from build123d import *

# Parameters (mm, degrees)
F1_DEPTH = 7.5
F3_DEPTH = 7.5
F4_SIZE  = 0.5


with BuildPart() as f1:
    # F0 (on Top) → F1 (new body, symmetric)
    with BuildSketch(Plane.XY):
        with BuildLine():
            ThreePointArc((16.7892444879, -0.9012567011), (14.177166416, 0), (16.7892444879, 0.9012567011))
            add(Edge.make_bspline(
                [(16.7892444879, 2.0751408301), (17.0817766167, 1.8643906524), (17.6043278119, 1.487926851), (17.1393225295, 0.8569863783), (16.895080973, 0.8878727844), (16.7892444879, 0.9012567011)],
                knots=[0, 0, 0, 0, 0.418834252, 0.7481651325, 1, 1, 1, 1], degree=3))
            ThreePointArc((16.7892444879, 2.0751408301), (13.2649986311, 0), (16.7892444879, -2.0751408301))
            add(Edge.make_bspline(
                [(16.7892444879, -2.0751408301), (17.0817766167, -1.8643906524), (17.6043278119, -1.487926851), (17.1393225295, -0.8569863783), (16.895080973, -0.8878727844), (16.7892444879, -0.9012567011)],
                knots=[0, 0, 0, 0, 0.418834252, 0.7481651325, 1, 1, 1, 1], degree=3))
        make_face()
    extrude(amount=F1_DEPTH, both=True)

    # F2 (on Top) → F3 (join, symmetric)
    with BuildSketch(Plane.XY):
        with BuildLine():
            ThreePointArc((11.4055118786, 1.0911012502), (12.1183137998, 0.8013586402), (12.4143324792, 0.0911401524))
            Line((12.4143324792, 0.0911401524), (12.4143324792, -0.0911401524))
            ThreePointArc((12.4143324792, -0.0911401524), (12.1183137998, -0.8013586402), (11.4055118786, -1.0911012502))
            Line((11.4055118786, -1.0911012502), (-10.2589782327, -0.9))
            Line((-10.2589782327, -0.9), (-10.2589782327, -2.1322260433))
            add(Edge.make_bspline(
                [(-10.2589782327, -2.1322260433), (-7.8308672605, -2.7680444958), (-2.1715241973, -4.4371278226), (14.2840922078, -4.2672083443), (14.5433608635, -2.4774637884), (14.5964084265, -2.1322260433)],
                knots=[0, 0, 0, 0, 0.3763600101, 0.8609680907, 1, 1, 1, 1], degree=3))
            Line((14.5964084265, -2.1322260433), (13.9306001365, -1.5301937237))
            Line((13.9306001365, -1.5301937237), (13.9306001365, 1.5301937237))
            Line((13.9306001365, 1.5301937237), (14.5964084265, 2.1322260433))
            add(Edge.make_bspline(
                [(-10.2589782327, 2.1322260433), (-7.8308672605, 2.7680444958), (-2.1715241973, 4.4371278226), (14.2840922078, 4.2672083443), (14.5433608635, 2.4774637884), (14.5964084265, 2.1322260433)],
                knots=[0, 0, 0, 0, 0.3763600101, 0.8609680907, 1, 1, 1, 1], degree=3))
            Line((-10.2589782327, 2.1322260433), (-10.2589782327, 0.9))
            Line((-10.2589782327, 0.9), (11.4055118786, 1.0911012502))
        make_face()
    extrude(amount=F3_DEPTH, both=True)

    # F4
    f4_edges = [f1.edges().sort_by_distance(p)[0] for p in [
        (-10.258978, -0.9, 0),
        (-10.258978, 0.9, 0),
    ]]
    chamfer(f4_edges, length=F4_SIZE)


solid = f1.part
Geometry check sheet. Reference: the model listing, model coordinates, mm. Give positions to 0.01 mm unless a question says otherwise; leave off trailing zeros. Answer in a Markdown table with one row per item. Add a question column.
1) Material ranges on probe 1 along Y at (x, z) = (8, -4.75); probe 2 along Y at (x, z) = (6, -3.25); probe 3 along Y at (x, z) = (12.75, -5.25), recorded low to high. Write a range as from..to.
2) Draft check along Y on faces 1 (the face through (12.11, 0.81, 0.11)), 2 (the face through (3, 2, -7.5)), 3 (the face through (12.13, -0.79, 0.11)). Enter one of: pulls with the +Y half, pulls with the -Y half, needs draft (parallel to the pull), parting line crosses it, or undercut.
3) Gauge pin test, flat ends, axial feed: P1, Ø2.5, axis at x = 15.64, y = 0, coming from the -Z side; P2, Ø3, axis at x = -7.5, z = 6, coming from the +Y side; P3, Ø8, axis at x = -5, z = -1, coming from the -Y side. Record the tip position at first contact, or that the pin passes through.
Outcome:
| question | item | result |
|---|---|---|
| 1 | probe 1 | y = -4.12..-1.06, 1.06..4.12 |
| 1 | probe 2 | y = -4.17..-1.04, 1.04..4.17 |
| 1 | probe 3 | y = -3.6..3.6 |
| 2 | face 1 | undercut |
| 2 | face 2 | needs draft |
| 2 | face 3 | undercut |
| 3 | P1 | passes through |
| 3 | P2 | stops at y = 3.18 |
| 3 | P3 | stops at y = -3.9 |
